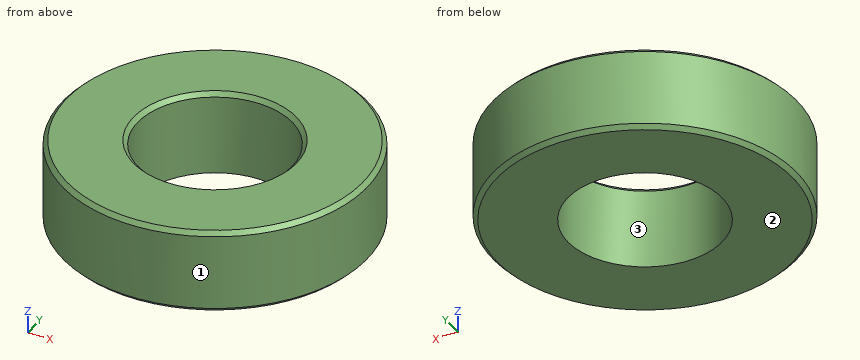
from build123d import *

# Parameters (mm, degrees)
F1_R     = 36.388832
F1_R_2   = 18.497226
F2_DEPTH = 20
F3_SIZE  = 1
F4_SIZE  = 1


with BuildPart() as f2:
    # F1 (on face) → F2 (new body)
    with BuildSketch(Plane.XY):
        Circle(F1_R)
        Circle(F1_R_2, mode=Mode.SUBTRACT)
    extrude(amount=F2_DEPTH)

    # F3
    f3_edges = [f2.edges().sort_by_distance(p)[0] for p in [
        (-36.388832, 0, 20),
        (-36.388832, 0, 0),
    ]]
    chamfer(f3_edges, length=F3_SIZE)

    # F4
    f4_edges = [f2.edges().sort_by_distance(p)[0] for p in [
        (-18.497226, 0, 20),
    ]]
    chamfer(f4_edges, length=F4_SIZE)


solid = f2.part
For this review, take the finished solid that the model builds, in its own axes (mm). Face numbers are marked on the shaded views. Give positions to 0.01 mm unless a question says otherwise; leave off trailing zeros. Loops run counter-clockwise (first coordinate to the right, second up) from the corner with the lowest first, then second, coordinate; pieces in that order, holes last. Notation, with made-up numbers: M -36.75,60 L -7.75,60 A12 ccw -7.75,74 Z; hole C -17.5,82.5 d2. An arc over 180 degrees is marked long. Answer as a JSON object with one key per item and string values. Group by question number.
Q1. For probe 1 along Y at (x, z) = (0, 6); probe 2 along Y at (x, z) = (11, 17.25); probe 3 along Y at (x, z) = (30, 5.5), list the stretches that pass through material, from the lowest coordinate up. Write a range as [from, to].
Q2. Add section C-C on z = 12. Give the boundary of the cut face in (x, y).
Q3. Insertion check: P1, Ø12, axis at y = -15.5, z = 14.5, coming from the -X side; P2, Ø8, axis at x = 2.5, z = 2.5, coming from the -Y side; P3, Ø8, axis at y = 14, z = 11.5, coming from the -X side. Each pin has a flat end and moves straight along its axis. Give the tip position at first contact, or say it passes through.
Q4. Mouldability with a two-part tool opening along X and no side actions: class the marked faces 1, 2 and 3 as +X half, -X half, draft (parallel to the pull), parting line (faces both ways), or undercut.
Q5. Add section A-A on y = 0. Give the boundary of the cut face in (x, z).
Checked values:
{
 "1": {"probe 1": "[-36.39, -18.5], [18.5, 36.39]", "probe 2": "[-34.69, -14.87], [14.87, 34.69]", "probe 3": "[-20.59, 20.59]"},
 "2": {"outline": "C 0,0 d72.78; hole C 0,0 d36.99"},
 "3": {"P1": "x = -35.13", "P2": "y = -36.39", "P3": "x = -34.99"},
 "4": {"face 1": "parting line", "face 2": "draft", "face 3": "undercut"},
 "5": {"outline": "M -36.39,1 L -35.39,0 L -18.5,0 L -18.5,19 L -19.5,20 L -35.39,20 L -36.39,19 Z; M 18.5,0 L 35.39,0 L 36.39,1 L 36.39,19 L 35.39,20 L 19.5,20 L 18.5,19 Z"}
}
